Verification items for the finished model (mm, model axes). A direction names the side the tool comes from. Give positions to 0.01 mm unless a question says otherwise; leave off trailing zeros. Order: outer loops, then holes, each group sorted by start corner. A loop starts at its lowest first (then second) coordinate and runs counter-clockwise, first axis right, second up.
(1) Mould release check, pull along Z, two halves, no side actions. Record for faces 1 (the face through (-0.04, -11.76, 22.12)), 2 (the face through (0, -5, 0)), 3 (the face through (0, -9.122, 10)), 4 (the face through (2.5, -11, 8)): pulls with the +Z half, pulls with the -Z half, needs draft (parallel to the pull), parting line crosses it, or undercut.
(2) Scan lines: L1, parallel to Z at x = 1.75, y = -11.75; L2, parallel to Y at x = 0, z = 2.2; L3, parallel to Z at x = 2.25, y = 1.75. Record each from-to range of solid material in increasing order.
(3) Access from +Z, -Z, +X, -X, +Y, -Y to the whole of each face (thin tool, end or side, straight path). Record for faces 5 (the face through (-2.5, -11, 8)), 6 (the face through (0, -14.122, 7)), 7 (the face through (1.617, -0.67, 2.465)).
(4) Sectioned sample at C-C on z = 19.5. Record the cut outline in (x, y), plus the area to 3 significant figures.
(5) Sectioned sample at B-B on x = -0.5. Record the cut outline in (y, z).
(6) Gauge pin test, flat ends, axial feed: pin 1 (3.5 mm diameter, centred on y = -11.5, z = 15, fed in from +X); pin 2 (4 mm diameter, centred on x = -0.5, z = 10.5, fed in from +Y); pin 3 (6 mm diameter, centred on y = -10, z = 6.5, fed in from -X). Record the tip position at first contact, or that the pin passes through.
(7) Sectioned sample at D-D on z = 1.5. Record the cut outline in (x, y), plus the area to 3 significant figures.
(8) Sectioned sample at A-A on y = 0. Record the cut outline in (x, z).
```python
from build123d import *

# Parameters (mm, degrees)
ESBO_O1_R                = 1.75
RESSALTO_EXTRUS_O1_DEPTH = 5
ESBO_O2_R                = 1.75
RESSALTO_EXTRUS_O2_DEPTH = 5


with BuildPart() as part:
    # Esboço1 → Ressalto-extrusão1 (new body)
    with BuildSketch(Plane.XY):
        with BuildLine():
            Line((-2.5, -3.122498999), (-2.5, -9.122498999))
            Line((-2.5, -9.122498999), (2.5, -9.122498999))
            Line((2.5, -9.122498999), (2.5, -3.122498999))
            ThreePointArc((2.5, -3.122498999), (0, 4), (-2.5, -3.122498999))
        make_face()
        Circle(ESBO_O1_R, mode=Mode.SUBTRACT)
    extrude(amount=RESSALTO_EXTRUS_O1_DEPTH)

    # Esboço2 → Ressalto-extrusão2 (add)
    with BuildSketch(Plane.ZY.offset(2.5)):
        with BuildLine():
            Line((0, -9.122498999), (0, -14.122498999))
            Line((0, -14.122498999), (15, -14.122498999))
            ThreePointArc((15, -14.122498999), (22.122498999, -11.622498999), (15, -9.122498999))
            Line((15, -9.122498999), (0, -9.122498999))
        make_face()
        with Locations((18.122498999, -11.622498999)):
            Circle(ESBO_O2_R, mode=Mode.SUBTRACT)
    extrude(amount=-RESSALTO_EXTRUS_O2_DEPTH)


solid = part.part
```
Ans:
1. face 1: undercut
1. face 2: pulls with the -Z half
1. face 3: undercut
1. face 4: needs draft
2. L1: z = 0 to 16.38, 19.87 to 22.12
2. L2: y = -14.12 to -1.75, 1.75 to 4
2. L3: z = 0 to 5
3. face 5: +Z, -Z, -X, -Y
3. face 6: -Z, +X, -X, -Y
3. face 7: +Z, -Z
4. outline: (-2.5, -15.38) - (2.5, -15.38) - (2.5, -12.7) - (-2.5, -12.7) - close; (-2.5, -10.54) - (2.5, -10.54) - (2.5, -7.87) - (-2.5, -7.87) - close
4. area: 26.8 mm2
5. outline: (-14.12, 0) - (-1.68, 0) - (-1.68, 5) - (-9.12, 5) - (-9.12, 15) arc R4 ccw (long way) to (-14.12, 15) - close; (1.68, 0) - (3.97, 0) - (3.97, 5) - (1.68, 5) - close; hole circle Ø3.5 at (-11.62, 18.12)
6. pin 1: stops at x = 2.5
6. pin 2: stops at y = -9.12
6. pin 3: stops at x = -2.5
7. outline: (-2.5, -14.12) - (2.5, -14.12) - (2.5, -3.12) arc R4 ccw (long way) to (-2.5, -3.12) - close; hole circle Ø3.5 at (0, 0)
7. area: 92.6 mm2
8. outline: (-4, 0) - (-1.75, 0) - (-1.75, 5) - (-4, 5) - close; (1.75, 0) - (4, 0) - (4, 5) - (1.75, 5) - close
